Check sheet for the modelled part. Datum: model origin and axes. Units: mm. A direction names the side the tool comes from. Coordinates: 2 decimals unless noted, no trailing zeros. Write each loop counter-clockwise with the first axis right and the second up, starting at its lowest first coordinate (ties: lowest second). Pieces come first, ordered by that corner, then holes. Notation, with made-up numbers: (51, 36) -> (72, 36) arc R18 ccw to (72, 46) -> close; hole circle Ø10 at (42.25, 84.25). An arc over 180 degrees is marked (long way). One line per item, written item: value. Start each with the question number.
1) Sectioned sample at B-B on x = 10. Enter the section's corners in (y, z).
2) Sectioned sample at A-A on y = -13. Enter the section's corners in (x, z).
3) Sectioned sample at C-C on z = -11. Enter the section's corners in (x, y).
4) Gauge pin test, flat ends, axial feed: P1, Ø8, axis at y = -6, z = 9.5, coming from the -X side; P2, Ø2.5, axis at y = -18, z = 1, coming from the -X side; P3, Ø10, axis at y = -13.5, z = 9.5, coming from the +X side; P4, Ø1.1, axis at y = 0.5, z = 12, coming from the +X side. Record the tip position at first contact, or that the pin passes through.
5) Sectioned sample at D-D on z = 8. Enter the section's corners in (x, y).
6) Scan lines: line 1 along Y through (x, z) = (10, -16.25); line 2 along X through (y, z) = (-14.5, -15); line 3 along Y through (x, z) = (8, 13.5). Record each from-to range of solid material in increasing order. Write a range as [from, to].
7) Set-up check for faces 5 (the flat face through (20, -7, 2)), 6 (the flat face through (0, -13, 1)), 7 (the flat face through (-89, 1, 13)): record each of +Z, -Z, +X, -X, +Y, -Y from which the full face is reachable in a straight line by a thin tool's end or side.
8) Draft check along X on faces 1 (the cylindrical face through (5.23, -11.5, -12.32)), 2 (the flat face through (10, -13, 0)), 3 (the cylindrical face through (12.4, -14.8, -12.7)), 4 (the flat face through (10, -13, 3)). Enter one of: +X half, -X half, draft (parallel to the pull), parting line (faces both ways), or undercut.
```python
from build123d import *

# Parameters (mm, degrees)
SKETCH1_W                = 20
SKETCH1_H                = 23
BOSS_EXTRUDE1_DEPTH      = 3
SKETCH2_W                = 20
SKETCH2_H                = 3
BOSS_EXTRUDE2_DEPTH      = 20
SKETCH3_R                = 5
BOSS_EXTRUDE3_DEPTH      = 25
SKETCH4_R                = 3
CUT_EXTRUDE1_DEPTH       = 25
SKETCH5_W                = 23
SKETCH5_H                = 3
BOSS_EXTRUDE4_DEPTH      = 87
BOSS_EXTRUDE5_DEPTH      = 5
BOSS_EXTRUDE5_DEPTH_BACK = 2
BOSS_EXTRUDE5_START      = 11.5


with BuildPart() as part:
    # Sketch1 → Boss-Extrude1 (new body)
    with BuildSketch(Plane.XY):
        with Locations((10, -11.5)):
            Rectangle(SKETCH1_W, SKETCH1_H)
    extrude(amount=BOSS_EXTRUDE1_DEPTH)

    # Sketch2 → Boss-Extrude2 (add)
    with BuildSketch(Plane.XY.offset(3)):
        with Locations((10, -1.5)):
            Rectangle(SKETCH2_W, SKETCH2_H)
    extrude(amount=BOSS_EXTRUDE2_DEPTH)

    # Sketch3 → Boss-Extrude3 (add)
    with BuildSketch(Plane(origin=(0, 0, 0), x_dir=(-1, 0, 0), z_dir=(0, 0, -1))):
        with Locations((-10, -13)):
            Circle(SKETCH3_R)
    extrude(amount=BOSS_EXTRUDE3_DEPTH)

    # Sketch4 → Cut-Extrude1 (cut)
    with BuildSketch(Plane(origin=(0, 0, -25), x_dir=(-1, 0, 0), z_dir=(0, 0, -1))):
        with Locations((-10, -13)):
            Circle(SKETCH4_R)
    extrude(amount=-CUT_EXTRUDE1_DEPTH, mode=Mode.SUBTRACT)

    # Sketch5 → Boss-Extrude4 (add)
    with BuildSketch(Plane.ZY):
        with Locations((11.5, -1.5)):
            Rectangle(SKETCH5_W, SKETCH5_H)
    extrude(amount=BOSS_EXTRUDE4_DEPTH)

    # Sketch8 → Boss-Extrude5 (add, two sides: drawn at the far end of the back side and taken through both)
    with BuildSketch(Plane.XY.offset(BOSS_EXTRUDE5_START - BOSS_EXTRUDE5_DEPTH_BACK)):
        Polygon((-87, 0), (-87, 1), (-90.55, 1), (-90.55, 0), (-93.55, 0), (-93.55, 1.75), (-90.55, 1.75), (-86, 1.75), (-86, 0), align=None)
    extrude(amount=BOSS_EXTRUDE5_DEPTH + BOSS_EXTRUDE5_DEPTH_BACK)


solid = part.part
```
Answers:
1. outline: (-23, 0) -> (-18, 0) -> (-18, -25) -> (-16, -25) -> (-16, 0) -> (-10, 0) -> (-10, -25) -> (-8, -25) -> (-8, 0) -> (0, 0) -> (0, 23) -> (-3, 23) -> (-3, 3) -> (-23, 3) -> close
2. outline: (0, 0) -> (5, 0) -> (5, -25) -> (7, -25) -> (7, 0) -> (13, 0) -> (13, -25) -> (15, -25) -> (15, 0) -> (20, 0) -> (20, 3) -> (0, 3) -> close
3. outline: circle Ø10 at (10, -13); hole circle Ø6 at (10, -13)
4. P1: stops at x = -87
4. P2: stops at x = 0
4. P3: passes through
4. P4: stops at x = 20
5. outline: (-87, -3) -> (20, -3) -> (20, 0) -> (-87, 0) -> close
6. line 1: y = [-18, -16], [-10, -8]
6. line 2: x = [5.23, 7.4], [12.6, 14.77]
6. line 3: y = [-3, 0]
7. face 5: +Z, -Z, +X, +Y, -Y
7. face 6: +Z, -Z, -X, -Y
7. face 7: +Z, -Z, -Y
8. face 1: parting line
8. face 2: undercut
8. face 3: undercut
8. face 4: draft
